from build123d import *

# Parameters (mm, degrees)
SKETCH_1_W      = 130
SKETCH_1_H      = 350
SKETCH_1_R      = 1.3
SKETCH_1_R_2    = 2.5
EXTRUDE_1_DEPTH = 3


with BuildPart() as part:
    # 草圖1 → 填料-伸長1 (new body)
    with BuildSketch(Plane.XY):
        Rectangle(SKETCH_1_W, SKETCH_1_H)
        with Locations((-30, 48.75)):
            Circle(SKETCH_1_R, mode=Mode.SUBTRACT)
        with Locations((-10, 48.75)):
            Circle(SKETCH_1_R, mode=Mode.SUBTRACT)
        with Locations((10, 48.75)):
            Circle(SKETCH_1_R, mode=Mode.SUBTRACT)
        with Locations((30, 48.75)):
            Circle(SKETCH_1_R, mode=Mode.SUBTRACT)
        with Locations((-30, -48.75)):
            Circle(SKETCH_1_R, mode=Mode.SUBTRACT)
        with Locations((-10, -48.75)):
            Circle(SKETCH_1_R, mode=Mode.SUBTRACT)
        with Locations((10, -48.75)):
            Circle(SKETCH_1_R, mode=Mode.SUBTRACT)
        with Locations((30, -48.75)):
            Circle(SKETCH_1_R, mode=Mode.SUBTRACT)
        with Locations((-52, -162)):
            Circle(SKETCH_1_R_2, mode=Mode.SUBTRACT)
        with Locations((-52, -144)):
            Circle(SKETCH_1_R_2, mode=Mode.SUBTRACT)
        with Locations((52, -144)):
            Circle(SKETCH_1_R_2, mode=Mode.SUBTRACT)
        with Locations((52, -162)):
            Circle(SKETCH_1_R_2, mode=Mode.SUBTRACT)
        with Locations((52, 162)):
            Circle(SKETCH_1_R_2, mode=Mode.SUBTRACT)
        with Locations((52, 144)):
            Circle(SKETCH_1_R_2, mode=Mode.SUBTRACT)
        with Locations((-52, 162)):
            Circle(SKETCH_1_R_2, mode=Mode.SUBTRACT)
        with Locations((-52, 144)):
            Circle(SKETCH_1_R_2, mode=Mode.SUBTRACT)
        Polygon((-37.928932188, -64.375), (37.928932188, -64.375), (0, -102.303932188), align=None, mode=Mode.SUBTRACT)
        Polygon((-7.071067812, -109.375), (-45, -71.446067812), (-45, -147.303932188), align=None, mode=Mode.SUBTRACT)
        Polygon((0, -116.446067812), (37.928932188, -154.375), (-37.928932188, -154.375), align=None, mode=Mode.SUBTRACT)
        Polygon((7.071067812, -109.375), (45, -71.446067812), (45, -147.303932188), align=None, mode=Mode.SUBTRACT)
        Polygon((-37.928932188, 154.375), (37.928932188, 154.375), (0, 116.446067812), align=None, mode=Mode.SUBTRACT)
        Polygon((-45, 147.303932188), (-7.071067812, 109.375), (-45, 71.446067812), align=None, mode=Mode.SUBTRACT)
        Polygon((0, 102.303932188), (-37.928932188, 64.375), (37.928932188, 64.375), align=None, mode=Mode.SUBTRACT)
        Polygon((7.071067812, 109.375), (45, 147.303932188), (45, 71.446067812), align=None, mode=Mode.SUBTRACT)
    extrude(amount=EXTRUDE_1_DEPTH)


solid = part.part
For this review, take the finished solid that the model builds, in its own axes (mm). A direction names the side the tool comes from. Coordinates: 2 decimals unless noted, no trailing zeros. Loops run counter-clockwise (first coordinate to the right, second up) from the corner with the lowest first, then second, coordinate; pieces in that order, holes last. Notation, with made-up numbers: (83.5, 8) - (100.5, 8) arc R24 ccw to (100.5, 46) - close; hole circle Ø1 at (58.5, 20). An arc over 180 degrees is marked (long way). Return JSON: item names as keys, results as strings.
Item 1: For line 1 (X direction, y = 162, z = 0.9); line 2 (Y direction, x = -52, z = 1.6); line 3 (Y direction, x = -50, z = 1.85), list the stretches that pass through material, from the lowest coordinate up.
Determined:
{"line 1": "x = -65 to -54.5, -49.5 to 49.5, 54.5 to 65", "line 2": "y = -175 to -164.5, -159.5 to -146.5, -141.5 to 141.5, 146.5 to 159.5, 164.5 to 175", "line 3": "y = -175 to -163.5, -160.5 to -145.5, -142.5 to 142.5, 145.5 to 160.5, 163.5 to 175"}
Item 2: Take a section at C-C (x = 42). Give the boundary of the cut face in (y, z).
Determined:
{"outline": "(-175, 0) - (-144.3, 0) - (-144.3, 3) - (-175, 3) - close; (-74.45, 0) - (74.45, 0) - (74.45, 3) - (-74.45, 3) - close; (144.3, 0) - (175, 0) - (175, 3) - (144.3, 3) - close"}
Item 3: Take a section at A-A (x = 16.5). Give the boundary of the cut face in (y, z) (3 decimals).
Determined:
{"outline": "(-175, 0) - (-154.375, 0) - (-154.375, 3) - (-175, 3) - close; (-132.946, 0) - (-118.804, 0) - (-118.804, 3) - (-132.946, 3) - close; (-99.946, 0) - (-85.804, 0) - (-85.804, 3) - (-99.946, 3) - close; (-64.375, 0) - (64.375, 0) - (64.375, 3) - (-64.375, 3) - close; (85.804, 0) - (99.946, 0) - (99.946, 3) - (85.804, 3) - close; (118.804, 0) - (132.946, 0) - (132.946, 3) - (118.804, 3) - close; (154.375, 0) - (175, 0) - (175, 3) - (154.375, 3) - close"}
Item 4: Insertion check: pin 1 (3.5 mm diameter, centred on x = -10, y = -48.75, fed in from -Z). The pin has a flat end and moves straight along its axis. Give the tip position at first contact, or say it passes through.
Determined:
{"pin 1": "stops at z = 0"}
Item 5: Take a section at D-D (z = 0.9). State how many separate pieces and enclosed holes the cut face has, then the cut area to 3 significant figures.
Determined:
{"separate pieces": "1", "enclosed holes": "24", "area": "33,800 mm2"}
Item 6: Take a section at B-B (y = 93). Give the boundary of the cut face in (x, z), then the cut area to 3 significant figures.
Determined:
{"outline": "(-65, 0) - (-45, 0) - (-45, 3) - (-65, 3) - close; (-23.45, 0) - (-9.3, 0) - (-9.3, 3) - (-23.45, 3) - close; (9.3, 0) - (23.45, 0) - (23.45, 3) - (9.3, 3) - close; (45, 0) - (65, 0) - (65, 3) - (45, 3) - close", "area": "205 mm2"}
Item 7: For faces 1 (the flat face through (-1, 2, 0)), 2 (the flat face through (18.699, -135.145, 1.479)), list the 3-axis set-ups (+Z, -Z, +X, -X, +Y, -Y) from which the entire face can be reached by the end or side of a thin tool; tool diameter is ignored.
Determined:
{"face 1": "-Z, +X, -X, +Y, -Y", "face 2": "+Z, -Z"}
Item 8: Mouldability with a two-part tool opening along Y and no side actions: class faces 3 (the flat face through (-25.77, -90.676, 1.479)), 4 (the flat face through (-25.77, 90.676, 1.479)), 5 (the flat face through (-1, 2, 3)) as pulls with the +Y half, pulls with the -Y half, needs draft (parallel to the pull), parting line crosses it, or undercut.
Determined:
{"face 3": "undercut", "face 4": "undercut", "face 5": "needs draft"}
